Could you check a few things on this model? Use its own coordinates, in mm. Face numbers are marked on the shaded views. A direction names the side the tool comes from. Round coordinates to 2 decimals unless told otherwise and drop trailing zeros. Loops run counter-clockwise (first coordinate to the right, second up) from the corner with the lowest first, then second, coordinate; pieces in that order, holes last. Notation, with made-up numbers: M 48,-10.5 L 68,-10.5 A34 cw 68,26.5 Z; hole C 9,-6 d7. An arc over 180 degrees is marked long. One line per item, written item: value. Start each with the question number.
Q1. Which directions (+Z, -Z, +X, -X, +Y, -Y) give clear straight access to the entire face, cutting with the end or side of a thin tool? Please do the marked faces 1, 2, 3 and 4.
Q2. I'm going to push flat-ended pins straight in: pin 1 Ø2.5 at (y, z) = (1.5, 3) entering from +X; pin 2 Ø2 at (y, z) = (-4, 1.5) entering from -X; pin 3 Ø1 at (x, z) = (23, 3.5) entering from +Y. Where does each tip first touch, or does it pass through?
Q3. Please list where these lines run through material, in increasing order: line 1 along Y through (x, z) = (17, 1.35); line 2 along Y through (x, z) = (25, 1.9); line 3 along Z through (x, y) = (14.5, 0.25).
Q4. Imagine slicing it at C-C (x = 10). Please give me the cut outline in (y, z).
Q5. Thinking about a two-plate mould opening in X: for the marked faces 5, 6 and 7, which applies, released by +X, released by -X, zero draft, split by the parting line, or undercut?
Q6. Imagine slicing it at A-A (z = 5.75). Please give me the cut outline in (x, y).
Q7. Imagine slicing it at B-B (y = -3.25). Please give me the cut outline in (x, z), then the cut area to 3 significant figures.
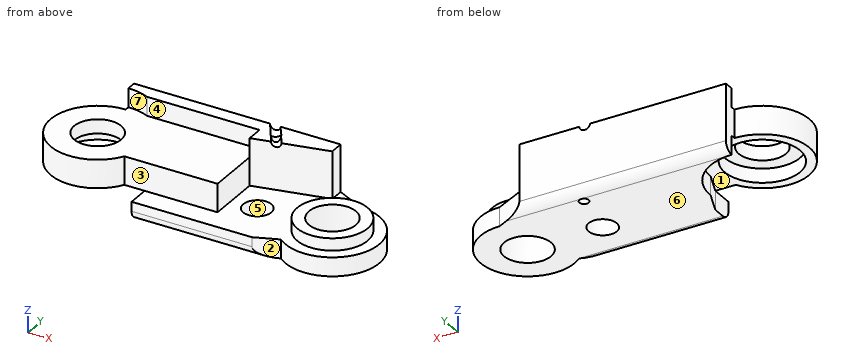
from build123d import *

# Parameters (mm, degrees)
BOSS_EXTRUDE1_DEPTH = 2
BOSS_EXTRUDE2_DEPTH = 5
BOSS_EXTRUDE3_DEPTH = 3
SKETCH7_R           = 2.5
CUT_EXTRUDE1_DEPTH  = 3
SKETCH8_R           = 4
CUT_EXTRUDE2_DEPTH  = 1.5
SKETCH12_R          = 3.75
BOSS_EXTRUDE5_DEPTH = 1.3
SKETCH13_R          = 2.5
CUT_EXTRUDE4_DEPTH  = 32.484122983
FILLET2_R           = 1
SKETCH14_R          = 1.5
CUT_EXTRUDE5_DEPTH  = 10
BOSS_EXTRUDE6_DEPTH = 5
SKETCH17_R          = 0.5
CUT_EXTRUDE6_DEPTH  = 32.484122983
SKETCH19_R          = 0.501737203
CUT_EXTRUDE7_DEPTH  = 5


with BuildPart() as part:
    # Sketch3 → Boss-Extrude1 (new body)
    with BuildSketch(Plane.XY):
        with BuildLine():
            Line((0, 5.5), (0, 6.5))
            Line((0, 6.5), (22, 6.5))
            Line((22, 6.5), (25, 5))
            ThreePointArc((25, 5), (29.704067696, -1.694623001), (21.811351474, -3.851301154))
            Line((21.811351474, -3.851301154), (19.311351474, -4.851301154))
            Line((19.311351474, -4.851301154), (6.5, -4.851301154))
            Line((6.5, -4.851301154), (6.5, -2.5))
            Line((6.5, -2.5), (5.5, 0))
            ThreePointArc((5.5, 0), (3.889087297, 3.889087297), (0, 5.5))
        make_face()
    extrude(amount=BOSS_EXTRUDE1_DEPTH)

    # Sketch4 → Boss-Extrude2 (add)
    with BuildSketch(Plane.XY.offset(2)):
        with BuildLine():
            Line((0, 6.5), (22, 6.5))
            Line((22, 6.5), (22, 5))
            Line((22, 5), (2.291287847, 5))
            ThreePointArc((2.291287847, 5), (1.17260394, 5.373546315), (0, 5.5))
            Line((0, 5.5), (0, 6.5))
        make_face()
    extrude(amount=BOSS_EXTRUDE2_DEPTH)

    # Sketch6 → Boss-Extrude3 (add)
    with BuildSketch(Plane.XY.offset(2)):
        with BuildLine():
            Line((2.291287847, 5), (12.145643924, 5))
            Line((12.145643924, 5), (14.255887023, 5))
            Line((14.255887023, 5), (14.255887023, -2.5))
            Line((14.255887023, -2.5), (12.145643924, -2.5))
            Line((12.145643924, -2.5), (6.5, -2.5))
            Line((6.5, -2.5), (4.330127019, -2.5))
            ThreePointArc((4.330127019, -2.5), (-4.330127019, -2.5), (0, 5))
            Line((0, 5), (0, 5.5))
            ThreePointArc((0, 5.5), (1.17260394, 5.373546315), (2.291287847, 5))
        make_face()
    extrude(amount=BOSS_EXTRUDE3_DEPTH)

    # Sketch7 → Cut-Extrude1 (cut)
    with BuildSketch(Plane(origin=(0, 0, 2), x_dir=(-1, 0, 0), z_dir=(0, 0, -1))):
        Circle(SKETCH7_R)
    extrude(amount=-CUT_EXTRUDE1_DEPTH, mode=Mode.SUBTRACT)

    # Sketch8 → Cut-Extrude2 (cut)
    with BuildSketch(Plane(origin=(0, 0, 2), x_dir=(-1, 0, 0), z_dir=(0, 0, -1))):
        Circle(SKETCH8_R)
    extrude(amount=-CUT_EXTRUDE2_DEPTH, mode=Mode.SUBTRACT)

    # Sketch12 → Boss-Extrude5 (add)
    with BuildSketch(Plane.XY.offset(2)):
        with Locations((25, 0)):
            Circle(SKETCH12_R)
    extrude(amount=BOSS_EXTRUDE5_DEPTH)

    # Sketch13 → Cut-Extrude4 (cut, through all)
    with BuildSketch(Plane(origin=(0, 0, 0), x_dir=(-1, 0, 0), z_dir=(0, 0, -1))):
        with Locations((-25, 0)):
            Circle(SKETCH13_R)
    extrude(amount=-CUT_EXTRUDE4_DEPTH, mode=Mode.SUBTRACT)

    # Fillet2
    fillet2_edges = [part.edges().sort_by_distance(p)[0] for p in [
        (12.905675737, -4.851301154, 0),
        (11, 6.5, 0),
    ]]
    fillet(fillet2_edges, radius=FILLET2_R - 0.0001)  # a hair under: the kernel refuses the full size

    # Sketch14 → Cut-Extrude5 (cut)
    with BuildSketch(Plane(origin=(0, 0, 0), x_dir=(-1, 0, 0), z_dir=(0, 0, -1))):
        with Locations((-17, 0)):
            Circle(SKETCH14_R)
    extrude(amount=-CUT_EXTRUDE5_DEPTH, mode=Mode.SUBTRACT)

    # Sketch16 → Boss-Extrude6 (add)
    with BuildSketch(Plane.XY.offset(2)):
        Polygon((14.255887023, 5), (14.255887023, 3.237297895), (22, 5), align=None)
    extrude(amount=BOSS_EXTRUDE6_DEPTH)

    # Sketch17 → Cut-Extrude6 (cut, through all)
    with BuildSketch(Plane.XY.offset(7)):
        with Locations((16, 5)):
            Circle(SKETCH17_R)
    extrude(amount=-CUT_EXTRUDE6_DEPTH, mode=Mode.SUBTRACT)

    # Sketch19 → Cut-Extrude7 (cut, along a direction that is not the sketch's normal)
    with BuildSketch(Plane(origin=(0.001645419, -0.007228852, 0), x_dir=(0.9750599765095712, 0.2219415288069236, 0), z_dir=(0.2219415288069236, -0.9750599765095712, 0))):
        with Locations((17.181227497, 7)):
            Circle(SKETCH19_R)
    extrude(amount=-CUT_EXTRUDE7_DEPTH, dir=(0.5357888185412162, -0.8443520248842943, 0), mode=Mode.SUBTRACT)


solid = part.part
Report:
1. face 1: -Z, -X, -Y
1. face 2: +Z, -Z, -Y
1. face 3: +Z, -Y
1. face 4: +Z, -X, -Y
2. pin 1: stops at x = 29.94
2. pin 2: stops at x = -3.9
2. pin 3: stops at y = 3.42
3. line 1: y = -4.85 to -1.5, 1.5 to 6.5
3. line 2: y = -5 to -2.5, 2.5 to 5
3. line 3: z = 0 to 2
4. outline: M -4.85,1 A1 ccw -3.85,0 L 5.5,0 A1 ccw 6.5,1 L 6.5,7 L 5,7 L 5,5 L -2.5,5 L -2.5,2 L -4.85,2 Z
5. face 5: undercut
5. face 6: zero draft
5. face 7: released by -X
6. outline: M 0,5.5 A5.5 cw 2.29,5 L 14.26,5 L 14.26,3.24 L 22,5 L 22,6.5 L 0,6.5 Z; hole C 16,5 d1
7. outline: M -3.8,2 L -2.33,2 L -2.33,3.5 L 2.33,3.5 L 2.33,2 L 3.8,2 L 3.8,5 L -3.8,5 Z; M 6.5,0 L 28.8,0 L 28.8,2 L 26.87,2 L 26.87,3.3 L 23.13,3.3 L 23.13,2 L 6.5,2 Z
7. area: 65.3 mm²
